Geometry check sheet. Reference: the model listing, model coordinates, mm. Round coordinates to 2 decimals unless told otherwise and drop trailing zeros. Order: outer loops, then holes, each group sorted by start corner. A loop starts at its lowest first (then second) coordinate and runs counter-clockwise, first axis right, second up. Notation, with made-up numbers: (11, 14.5) - (68, 14.5) arc R14 ccw to (68, 40.5) - close; hole circle Ø10 at (36, 40.25). An arc over 180 degrees is marked (long way). Write each question's results on one line, items separated by ' | '.
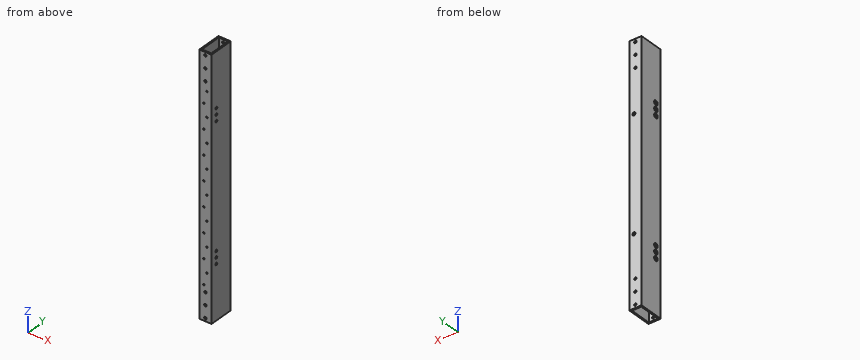
```python
from build123d import *

# Parameters (mm, degrees)
SKETCH1_W                                       = 25.4
SKETCH1_H                                       = 50.8
SKETCH1_W_2                                     = 19.05
SKETCH1_H_2                                     = 44.45
EXTRUDE_THIN1_DEPTH                             = 527.05
F_10_CLEARANCE_HOLE1_D                          = 5.1054
F_1_8_0_13_DIAMETER_HOLE1_D                     = 3.302
F_1_8_0_13_DIAMETER_HOLE1_DEPTH                 = 3.175
F_1_4_0_25_DIAMETER_HOLE1_D                     = 6.35
F_1_4_0_25_DIAMETER_HOLE1_DEPTH                 = 10.7188
F_1_4_0_25_DIAMETER_HOLE1_TIP                   = 1.907732465
CBORE_FOR_10_SOCKET_HEAD_CAP_SCREW1_D           = 5.1054
CBORE_FOR_10_SOCKET_HEAD_CAP_SCREW1_CBORE_D     = 9.525
CBORE_FOR_10_SOCKET_HEAD_CAP_SCREW1_CBORE_DEPTH = 8.001


with BuildPart() as part:
    # Sketch1 → Extrude-Thin1 (new body)
    with BuildSketch(Plane.XY):
        Rectangle(SKETCH1_W, SKETCH1_H)
        Rectangle(SKETCH1_W_2, SKETCH1_H_2, mode=Mode.SUBTRACT)
    extrude(amount=EXTRUDE_THIN1_DEPTH)

    # #10 Clearance Hole1 (through all)
    with Locations(Plane(origin=(0, 25.4, 0), x_dir=(1, 0, 0), z_dir=(0, 1, 0))):
        with Locations((0, -520.7), (0, -495.3), (0, -469.9), (0, -6.35), (0, -31.75), (0, -57.15)):
            Hole(F_10_CLEARANCE_HOLE1_D / 2)

    # 1/8 (0.13) Diameter Hole1
    with Locations(Plane(origin=(0, -25.4, 0), x_dir=(-1, 0, 0), z_dir=(0, -1, 0))):
        with Locations((3.175, -70.358), (-3.175, -95.758), (3.175, -121.158), (-3.175, -146.558), (3.175, -171.958), (-3.175, -197.358), (-3.175, -248.158), (3.175, -273.558), (-3.175, -298.958), (3.175, -324.358), (-3.175, -349.758), (3.175, -375.158), (-3.175, -400.558), (3.175, -425.958), (-3.175, -451.358), (3.175, -222.758)):
            Hole(F_1_8_0_13_DIAMETER_HOLE1_D / 2, depth=F_1_8_0_13_DIAMETER_HOLE1_DEPTH)

    # 1/4 (0.25) Diameter Hole1
    with Locations(Plane(origin=(0, 25.4, 0), x_dir=(1, 0, 0), z_dir=(0, 1, 0))):
        with Locations((3.175, -146.05), (3.175, -381)):
            Hole(F_1_4_0_25_DIAMETER_HOLE1_D / 2, depth=F_1_4_0_25_DIAMETER_HOLE1_DEPTH)
            with Locations((0, 0, -(F_1_4_0_25_DIAMETER_HOLE1_DEPTH + F_1_4_0_25_DIAMETER_HOLE1_TIP / 2))):  # 118° drill point
                Cone(0, F_1_4_0_25_DIAMETER_HOLE1_D / 2, F_1_4_0_25_DIAMETER_HOLE1_TIP, mode=Mode.SUBTRACT)

    # CBORE for #10 Socket Head Cap Screw1 (through all)
    with Locations(Plane.ZY.offset(12.7)):
        with Locations((111.125, -12.7), (123.825, -12.7), (136.525, -12.7), (390.525, -12.7), (403.225, -12.7), (415.925, -12.7)):
            CounterBoreHole(CBORE_FOR_10_SOCKET_HEAD_CAP_SCREW1_D / 2, CBORE_FOR_10_SOCKET_HEAD_CAP_SCREW1_CBORE_D / 2, CBORE_FOR_10_SOCKET_HEAD_CAP_SCREW1_CBORE_DEPTH)


solid = part.part
```
(1) Section check A-A (y = 2.5). Record the cut outline in (x, z) (3 decimals).
Answers follow:
outline: (-12.7, 0) - (-9.525, 0) - (-9.525, 527.05) - (-12.7, 527.05) - close; (9.525, 0) - (12.7, 0) - (12.7, 527.05) - (9.525, 527.05) - close
(2) Depth check by flat-ended pin: pin 1 Ø2.5 at (x, z) = (3.175, 248.158) entering from -Y (3 decimals); pin 2 Ø12 at (x, y) = (-2.5, 7.5) entering from -Z. Enter the tip coordinate at first touch or a pass-through.
Answers follow:
pin 1: y = 22.225 | pin 2: through
(3) Section check B-B (z = 213). Record the cut outline in (x, y) (3 decimals).
Answers follow:
outline: (-12.7, -25.4) - (12.7, -25.4) - (12.7, 25.4) - (-12.7, 25.4) - close; hole (-9.525, -22.225) - (9.525, -22.225) - (9.525, 22.225) - (-9.525, 22.225) - close
(4) Material ranges on line 1 (Y direction, x = -6.25, z = 339.5) (3 decimals); line 2 (X direction, y = -6.5, z = 464.5) (3 decimals); line 3 (X direction, y = -23, z = 6), recorded low to high.
Answers follow:
line 1: -25.4 to -22.225, 22.225 to 25.4 | line 2: -12.7 to -9.525, 9.525 to 12.7 | line 3: -12.7 to -2.53, 2.53 to 12.7
